```python
from build123d import *

# Parameters (mm, degrees)
SKETCH1_R           = 2.0193
SKETCH1_R_2         = 14.478
SKETCH1_R_3         = 2.6289
BOSS_EXTRUDE1_DEPTH = 6.35


with BuildPart() as part:
    # Sketch1 → Boss-Extrude1 (new body)
    with BuildSketch(Plane(origin=(0, 0, 0), x_dir=(1, 0, 0), z_dir=(0, 1, 0))):
        with BuildLine():
            Line((-313.888905321, 171.087609001), (-222.249489346, 171.087609001))
            Line((-222.249489346, 171.087609001), (-222.249489346, 145.888937334))
            Line((-222.249489346, 145.888937334), (-261.213202804, 100.464511352))
            ThreePointArc((-261.213202804, 100.464511352), (-265.91335193, 97.482933567), (-271.477290762, 97.637181964))
            Line((-271.477290762, 97.637181964), (-293.038636115, 104.883600221))
            ThreePointArc((-293.038636115, 104.883600221), (-301.131013118, 109.898805053), (-306.14621795, 117.991182056))
            Line((-306.14621795, 117.991182056), (-313.392636207, 139.552527409))
            ThreePointArc((-313.392636207, 139.552527409), (-313.764019328, 141.049575419), (-313.888905321, 142.586937334))
            Line((-313.888905321, 142.586937334), (-313.888905321, 171.087609001))
        make_face()
        with Locations((-228.599489346, 158.427874667)):
            Circle(SKETCH1_R, mode=Mode.SUBTRACT)
        with Locations((-241.299425514, 158.387609001)):
            Circle(SKETCH1_R, mode=Mode.SUBTRACT)
        with Locations((-253.999361682, 158.347343334)):
            Circle(SKETCH1_R, mode=Mode.SUBTRACT)
        with Locations((-266.69929785, 158.307077667)):
            Circle(SKETCH1_R, mode=Mode.SUBTRACT)
        with Locations((-279.399234018, 158.266812001)):
            Circle(SKETCH1_R, mode=Mode.SUBTRACT)
        with Locations((-292.099170186, 158.226546334)):
            Circle(SKETCH1_R, mode=Mode.SUBTRACT)
        with Locations((-304.799106355, 158.186280667)):
            Circle(SKETCH1_R, mode=Mode.SUBTRACT)
        with Locations((-286.403393079, 124.626425091)):
            Circle(SKETCH1_R_2, mode=Mode.SUBTRACT)
        with Locations((-268.442880837, 106.665912849)):
            Circle(SKETCH1_R_3, mode=Mode.SUBTRACT)
        with Locations((-304.363905321, 142.586937334)):
            Circle(SKETCH1_R_3, mode=Mode.SUBTRACT)
        with Locations((-241.299425514, 132.987609001)):
            Circle(SKETCH1_R, mode=Mode.SUBTRACT)
    extrude(amount=BOSS_EXTRUDE1_DEPTH)


solid = part.part
```
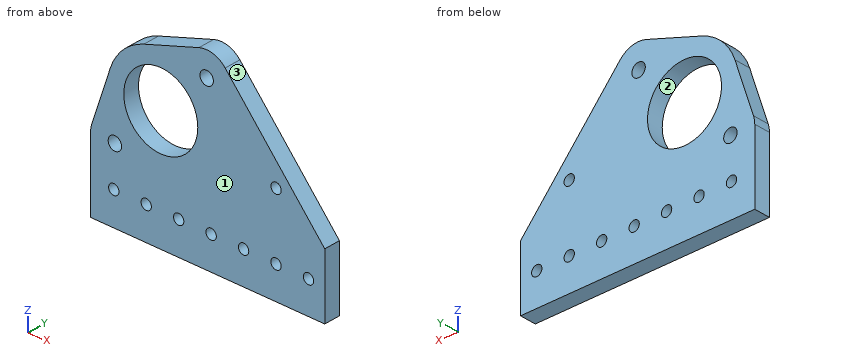
Geometry: final body of the model. Coordinates: model frame, mm. Face numbers are marked on the shaded views. Give positions to 0.01 mm unless a question says otherwise; leave off trailing zeros. Write each loop counter-clockwise with the first axis right and the second up, starting at its lowest first coordinate (ties: lowest second). Pieces come first, ordered by that corner, then holes.
1. Section query D-D, the plane z = -103. Return loops of the section in (x, y), then the cut area to 3 significant figures.
2. Section query A-A, the plane z = -121.5. Return loops of the section in (x, y).
3. Section query B-B, the plane y = 4.5. Count the separate pieces of the cut face and the enclosed holes in it, then the cut area to 3 significant figures.
4. Line query: probe 1 along Z at (x, y) = (-241.5, 1); probe 2 along Z at (x, y) = (-243, 5.25); probe 3 along Z at (x, y) = (-228.5, 1). Output: solid intervals per line, ascending.
5. Section query C-C, the plane x = -276. Return loops of the section in (y, z), then the cut area to 3 significant figures.
6. Pin query (flat end, axial travel): P1, Ø3.5, axis at x = -279.4, z = -158.27, coming from the +Y side; P2, Ø3, axis at y = 1, z = -123, coming from the -X side. Return the tip coordinate at first contact, or that it passes through.
7. Draft query along Z for the marked faces 1, 2 and 3. Return one class per face: released by +Z, released by -Z, zero draft, split by the parting line, or undercut.
Computed:
1. outline: (-287.43, 0) - (-259.04, 0) - (-259.04, 6.35) - (-287.43, 6.35) - close
1. area: 180 mm2
2. outline: (-307.33, 0) - (-300.54, 0) - (-300.54, 6.35) - (-307.33, 6.35) - close; (-272.27, 0) - (-243.17, 0) - (-243.17, 6.35) - (-272.27, 6.35) - close
3. separate pieces: 1
3. enclosed holes: 11
3. area: 4,450 mm2
4. probe 1: z = -171.09 to -160.4, -156.38 to -135, -130.98 to -123.45
4. probe 2: z = -171.09 to -159.48, -157.3 to -134.08, -131.9 to -121.7
4. probe 3: z = -171.09 to -160.44, -156.41 to -138.6
5. outline: (0, -171.09) - (6.35, -171.09) - (6.35, -134.7) - (0, -134.7) - close; (0, -114.56) - (6.35, -114.56) - (6.35, -99.16) - (0, -99.16) - close
5. area: 329 mm2
6. P1: passes through
6. P2: stops at x = -308.33
7. face 1: zero draft
7. face 2: undercut
7. face 3: released by +Z
